```python
from build123d import *

# Parameters (mm, degrees)
SKETCH1_W           = 101.6
SKETCH1_H           = 25.4
SKETCH1_R           = 6.35
SKETCH1_R_2         = 3.175
BOSS_EXTRUDE1_DEPTH = 25.4
SKETCH2_W           = 19.05
SKETCH2_H           = 19.05
CUT_EXTRUDE1_DEPTH  = 106.494123059


with BuildPart() as part:
    # Sketch1 → Boss-Extrude1 (new body)
    with BuildSketch(Plane(origin=(0, 0, 0), x_dir=(1, 0, 0), z_dir=(0, 1, 0))):
        with Locations((38.1, 0)):
            Rectangle(SKETCH1_W, SKETCH1_H)
        with Locations(Location((44.45, 0, 0), (0, 0, 270))):
            Circle(SKETCH1_R, mode=Mode.SUBTRACT)
        with Locations(Location((76.2, 0, 0), (0, 0, 270))):
            Circle(SKETCH1_R_2, mode=Mode.SUBTRACT)
        Polygon((7.332348419, 0), (3.666174209, 6.35), (-3.666174209, 6.35), (-7.332348419, 0), (-3.666174209, -6.35), (3.666174209, -6.35), align=None, mode=Mode.SUBTRACT)
    extrude(amount=BOSS_EXTRUDE1_DEPTH)

    # Sketch2 → Cut-Extrude1 (cut, through all)
    with BuildSketch(Plane(origin=(88.9, 0, 0), x_dir=(0, 0, -1), z_dir=(1, 0, 0))):
        with Locations((0, 12.7)):
            Rectangle(SKETCH2_W, SKETCH2_H)
    extrude(amount=-CUT_EXTRUDE1_DEPTH, mode=Mode.SUBTRACT)


solid = part.part
```
Work out the finished part from the listing and answer in its coordinate system (mm). A direction names the side the tool comes from. Give positions to 0.01 mm unless a question says otherwise; leave off trailing zeros. Loops run counter-clockwise (first coordinate to the right, second up) from the corner with the lowest first, then second, coordinate; pieces in that order, holes last. Notation, with made-up numbers: (88.5, 29) -> (111.5, 29) arc R11 ccw to (111.5, 45) -> close; hole circle Ø8 at (-24, -24.75). An arc over 180 degrees is marked (long way). Put each result on its own line as item: value. Start each with the question number.
Item 1: The part is cut by section C-C (z = 1.5). State how many separate pieces and enclosed holes the cut face has, then the cut area to 3 significant figures.
Item 2: The mould has two halves that part along Y. Classify faces 1 (the face through (0, 24, -6.35)), 2 (the face through (37, 25.4, 0)), 3 (the face through (39, 22.225, 4)): released by +Y, released by -Y, zero draft, split by the parting line, or undercut.
Item 3: Find the intervals of material crossed by L1, parallel to X at y = 1.2, z = 0 (3 decimals); L2, parallel to Z at x = 1, y = 10 (3 decimals); L3, parallel to Z at x = 76.2, y = 0.9 (3 decimals), in increasing order. Write a range as [from, to].
Item 4: The part is cut by section D-D (x = 37). Give the vertices of the cut face in (y, z) (3 decimals), then the cut area to 3 significant figures.
Item 5: The part is cut by section B-B (y = 20.75). Give the vertices of the cut face in (x, z) (3 decimals).
Item 6: Which of the six approach directions +Z, -Z, +X, -X, +Y, -Y give full straight-line access (tool end or side, diameter ignored) to faces 4 (the face through (-5.525, 23.79, 3.131)), 5 (the face through (39, 13, 9.525)), 6 (the face through (37, 13, 12.7))?
Item 7: Each of these flat-tipped pins is pushed along its axis until it touches: P1, Ø1.5, axis at x = 11, z = 1.5, coming from the -Y side; P2, Ø7.5, axis at x = 44.45, z = 0, coming from the -Y side. Where does it stop, or does it pass through?
Item 8: The part is cut by section A-A (x = 76.2). Give the vertices of the cut face in (y, z) (3 decimals).
Answers below:
1. separate pieces: 8
1. enclosed holes: 0
1. area: 449 mm2
2. face 1: zero draft
2. face 2: released by +Y
2. face 3: undercut
3. L1: [-12.7, -7.332], [7.332, 38.1], [50.8, 73.025], [79.375, 88.9]
3. L2: [-12.7, -9.525], [9.525, 12.7]
3. L3: [-12.7, -3.175], [3.175, 12.7]
4. outline: (0, -12.7) -> (25.4, -12.7) -> (25.4, 12.7) -> (0, 12.7) -> close; hole (3.175, -9.525) -> (22.225, -9.525) -> (22.225, 9.525) -> (3.175, 9.525) -> close
4. area: 282 mm2
5. outline: (-12.7, -12.7) -> (88.9, -12.7) -> (88.9, -9.525) -> (-12.7, -9.525) -> close; (-12.7, 9.525) -> (88.9, 9.525) -> (88.9, 12.7) -> (-12.7, 12.7) -> close
6. face 4: +Y, -Y
6. face 5: +X, -X
6. face 6: +Z, +X, -X, +Y, -Y
7. P1: y = 0
7. P2: through
8. outline: (0, -12.7) -> (25.4, -12.7) -> (25.4, -3.175) -> (22.225, -3.175) -> (22.225, -9.525) -> (3.175, -9.525) -> (3.175, -3.175) -> (0, -3.175) -> close; (0, 3.175) -> (3.175, 3.175) -> (3.175, 9.525) -> (22.225, 9.525) -> (22.225, 3.175) -> (25.4, 3.175) -> (25.4, 12.7) -> (0, 12.7) -> close
